Build history of the part. All positions in model axes, mm. A direction names the side the tool comes from. Coordinates: 2 decimals unless noted, no trailing zeros. Order: outer loops, then holes, each group sorted by start corner. A loop starts at its lowest first (then second) coordinate and runs counter-clockwise, first axis right, second up. Notation, with made-up numbers: M -35.75,4 L 9.25,4 A15 cw 9.25,13 Z; hole C -35.75,62.25 d1. An arc over 180 degrees is marked long. Write item = value, one per line. Start each with the question number.
Q1. Band-saw the part on B-B on x = 36.5. Write the cut outline in (y, z).
Q2. Band-saw the part on A-A on y = 57.5. Write the cut outline in (x, z), plus the area to 3 significant figures.
Q3. Pull direction Y, two halves, no side cores. Call faces 4 (the face through (41, 191, 3)), 5 (the face through (49.967, 53, 3)), 6 (the face through (41.348, -23.003, 1.479)): released by +Y, released by -Y, zero draft, split by the parting line, or undercut.
Q4. Drill centre lines: probe 1 along Y at (x, z) = (41.75, 2.65); probe 2 along Y at (x, z) = (40.25, 3.2); probe 3 along X at (y, z) = (116.5, 0.65). Where is each one in solid material? Low to high.
Q5. Pin check, flat tips, straight feed: P1, Ø14, axis at x = 48, y = 197.5, coming from the -Z side; P2, Ø2, axis at x = 31, z = 5.5, coming from the +Y side. Stop position of each tip, or through.
Q6. Band-saw the part on C-C on z = 1.85. Write the cut outline in (x, y) (3 decimals), plus the area to 3 significant figures.
Q7. Band-saw the part on D-D on y = 93. Write the cut outline in (x, z), plus the area to 3 significant figures.
Q8. 3-axis set-ups, long thin cutter, end or side, ignore diameter. For faces 1 (the face through (40.846, 149.842, 3.042)), 2 (the face through (41.348, 176.997, 1.479)), 3 (the face through (41, -9, 3)): which of +Z, -Z, +X, -X, +Y, -Y reach the whole face in a straight line?
```python
from build123d import *

# Parameters (mm, degrees)
ESQUISSE1_W             = 27.85
ESQUISSE1_H             = 200
BOSS_EXTRU_1_DEPTH      = 6
ESQUISSE2_R             = 13.925
ENL_V_MAT_EXTRU_1_DEPTH = 3
ESQUISSE3_R             = 13.925
ENL_V_MAT_EXTRU_2_DEPTH = 3
ESQUISSE5_W             = 17.85
ESQUISSE5_H             = 25
ESQUISSE5_R             = 8.925
ENL_V_MAT_EXTRU_3_DEPTH = 10


with BuildPart() as part:
    # Esquisse1 → Boss.-Extru.1 (new body)
    with BuildSketch(Plane.XY):
        with Locations((41.042105263, 90.919078947)):
            Rectangle(ESQUISSE1_W, ESQUISSE1_H)
        with BuildLine():
            Line((27.117105263, -9.080921053), (54.967105263, -9.080921053))
            ThreePointArc((54.967105263, -9.080921053), (41.042105263, -23.005921053), (27.117105263, -9.080921053))
        make_face()
        with BuildLine():
            ThreePointArc((27.117105263, 190.919078947), (41.042105263, 204.844078947), (54.967105263, 190.919078947))
            Line((54.967105263, 190.919078947), (27.117105263, 190.919078947))
        make_face()
    extrude(amount=BOSS_EXTRU_1_DEPTH)

    # Esquisse2 → Enlèv. mat.-Extru.1 (cut)
    with BuildSketch(Plane.XY.offset(6)):
        with Locations((41.042105263, -9.080921053)):
            Circle(ESQUISSE2_R)
    extrude(amount=-ENL_V_MAT_EXTRU_1_DEPTH, mode=Mode.SUBTRACT)

    # Esquisse3 → Enlèv. mat.-Extru.2 (cut)
    with BuildSketch(Plane(origin=(0, 0, 0), x_dir=(-1, 0, 0), z_dir=(0, 0, -1))):
        with Locations((-41.042105263, 190.919078947)):
            Circle(ESQUISSE3_R)
    extrude(amount=-ENL_V_MAT_EXTRU_2_DEPTH, mode=Mode.SUBTRACT)

    # Esquisse5 → Enlèv. mat.-Extru.3 (cut)
    with BuildSketch(Plane.XY.offset(6)):
        with BuildLine():
            ThreePointArc((32.117105263, 140.919078947), (41.042105263, 149.844078947), (49.967105263, 140.919078947))
            Line((49.967105263, 140.919078947), (32.117105263, 140.919078947))
        make_face()
        with Locations((41.042105263, 128.419078947)):
            Rectangle(ESQUISSE5_W, ESQUISSE5_H)
        with BuildLine():
            ThreePointArc((49.967105263, 115.919078947), (41.042105263, 106.994078947), (32.117105263, 115.919078947))
            Line((32.117105263, 115.919078947), (49.967105263, 115.919078947))
        make_face()
        with Locations((41.042105263, 90.919078947)):
            Circle(ESQUISSE5_R)
        with BuildLine():
            ThreePointArc((32.117105263, 65.919078947), (41.042105263, 74.844078947), (49.967105263, 65.919078947))
            Line((49.967105263, 65.919078947), (32.117105263, 65.919078947))
        make_face()
        with Locations((41.042105263, 53.419078947)):
            Rectangle(ESQUISSE5_W, ESQUISSE5_H)
        with BuildLine():
            Line((32.117105263, 40.919078947), (49.967105263, 40.919078947))
            ThreePointArc((49.967105263, 40.919078947), (41.042105263, 31.994078947), (32.117105263, 40.919078947))
        make_face()
        with Locations((41.042105263, 15.919078947)):
            Circle(ESQUISSE5_R)
    extrude(amount=-ENL_V_MAT_EXTRU_3_DEPTH, mode=Mode.SUBTRACT)


solid = part.part
```
Recorded:
q1.outline = M -22.24,0 L 8.24,0 L 8.24,6 L 4.08,6 L 4.08,3 L -22.24,3 Z; M 23.6,0 L 33.24,0 L 33.24,6 L 23.6,6 Z; M 73.6,0 L 83.24,0 L 83.24,6 L 73.6,6 Z; M 98.6,0 L 108.24,0 L 108.24,6 L 98.6,6 Z; M 148.6,0 L 177.76,0 L 177.76,3 L 204.08,3 L 204.08,6 L 148.6,6 Z
q2.outline = M 27.12,0 L 32.12,0 L 32.12,6 L 27.12,6 Z; M 49.97,0 L 54.97,0 L 54.97,6 L 49.97,6 Z
q2.area = 60.0 mm2
q3.face_4 = zero draft
q3.face_5 = undercut
q3.face_6 = released by -Y
q4.probe_1 = -22.99 to 7.02, 24.82 to 32.02, 74.82 to 82.02, 99.82 to 107.02, 149.82 to 177.01
q4.probe_2 = 4.82 to 7.03, 24.81 to 32.03, 74.81 to 82.03, 99.81 to 107.03, 149.81 to 204.82
q4.probe_3 = 27.12 to 32.12, 49.97 to 54.97
q5.P1 = 3
q5.P2 = 201.51
q6.outline = M 27.117,-9.081 A13.925 ccw 54.967,-9.081 L 54.967,190.919 A13.925 cw 27.117,190.919 Z; hole C 41.042,15.919 d17.85; hole M 32.117,40.919 A8.925 ccw 49.967,40.919 L 49.967,65.919 A8.925 ccw 32.117,65.919 Z; hole C 41.042,90.919 d17.85; hole M 32.117,115.919 A8.925 ccw 49.967,115.919 L 49.967,140.919 A8.925 ccw 32.117,140.919 Z
q6.area = 3,680 mm2
q7.outline = M 27.12,0 L 32.36,0 L 32.36,6 L 27.12,6 Z; M 49.72,0 L 54.97,0 L 54.97,6 L 49.72,6 Z
q7.area = 63.0 mm2
q8.face_1 = +Z, -Z
q8.face_2 = -Z, +Y
q8.face_3 = +Z, -Y
